from build123d import *

# Parameters (mm, degrees)
ESQUISSE1_R        = 2
BOSS_EXTRU_1_DEPTH = 6


with BuildPart() as part:
    # Esquisse1 → Boss.-Extru.1 (new body)
    with BuildSketch(Plane.XY):
        with BuildLine():
            Line((0, 0), (0, 26.7))
            ThreePointArc((0, 26.7), (10, 36.7), (20, 26.7))
            Line((20, 26.7), (20, 12))
            Line((20, 12), (17, 12))
            Line((17, 12), (17, 6))
            Line((17, 6), (15.05, 6))
            Line((15.05, 6), (15.05, 0))
            Line((15.05, 0), (10, 0))
            Line((10, 0), (10, 6))
            Line((10, 6), (5.05, 6))
            Line((5.05, 6), (5.05, 0))
            Line((5.05, 0), (0, 0))
        make_face()
        with Locations((10, 26.7)):
            Circle(ESQUISSE1_R, mode=Mode.SUBTRACT)
    extrude(amount=BOSS_EXTRU_1_DEPTH)


solid = part.part
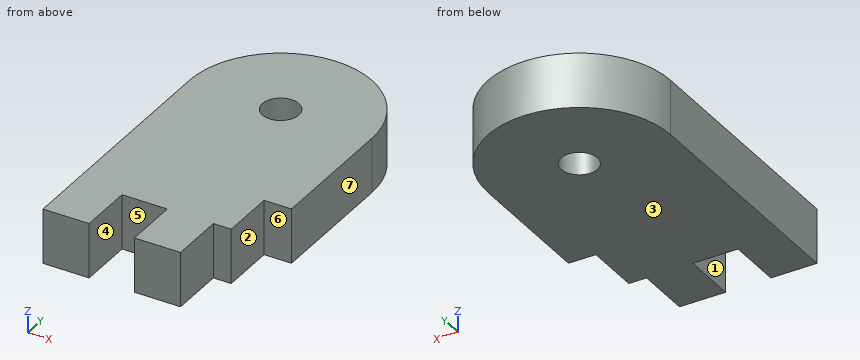
Verification items for the finished model (mm, model axes). Face numbers are marked on the shaded views. A direction names the side the tool comes from. Coordinates: 2 decimals unless noted, no trailing zeros. Order: outer loops, then holes, each group sorted by start corner. A loop starts at its lowest first (then second) coordinate and runs counter-clockwise, first axis right, second up.
Item 1: Release check for a two-part mould opening along X. For the marked faces 1, 2, 3 and 4 record: +X half, -X half, draft (parallel to the pull), parting line (faces both ways), or undercut.
Filled in:
face 1: undercut
face 2: +X half
face 3: draft
face 4: undercut
Item 2: Depth check by flat-ended pin: pin 1 (1.6 mm diameter, centred on x = 16.5, z = 3.5, fed in from -Y); pin 2 (3 mm diameter, centred on y = 1.5, z = 3, fed in from +X); pin 3 (1.5 mm diameter, centred on y = 29.5, z = 4.5, fed in from +X). Enter the tip coordinate at first touch or a pass-through.
Filled in:
pin 1: stops at y = 6
pin 2: stops at x = 15.05
pin 3: stops at x = 19.79
Item 3: Material ranges on L1, parallel to X at y = 5.5, z = 2.25; L2, parallel to X at y = 6.5, z = 3.15; L3, parallel to Y at x = 9.25, z = 0.3, recorded low to high.
Filled in:
L1: x = 0 to 5.05, 10 to 15.05
L2: x = 0 to 17
L3: y = 6 to 24.85, 28.55 to 36.67
Item 4: Section check A-A, the plane z = 3. Enter the section's corners in (x, y), then the cut area to 3 significant figures.
Filled in:
outline: (0, 0) - (5.05, 0) - (5.05, 6) - (10, 6) - (10, 0) - (15.05, 0) - (15.05, 6) - (17, 6) - (17, 12) - (20, 12) - (20, 26.7) arc R10 ccw to (0, 26.7) - close; hole circle Ø4 at (10, 26.7)
area: 601 mm2
Item 5: Access from +Z, -Z, +X, -X, +Y, -Y to the whole of each face (thin tool, end or side, straight path). Record for the marked faces 5, 6 and 7.
Filled in:
face 5: +Z, -Z, -Y
face 6: +Z, -Z, +X, -Y
face 7: +Z, -Z, +X, +Y, -Y
Item 6: Section check B-B, the plane y = 10. Enter the section's corners in (x, z).
Filled in:
outline: (0, 0) - (17, 0) - (17, 6) - (0, 6) - close
Item 7: Section check C-C, the plane x = 5.75. Enter the section's corners in (y, z).
Filled in:
outline: (6, 0) - (35.75, 0) - (35.75, 6) - (6, 6) - close
